Can you work these out from the model? Positions are in its coordinate system, mm. Round coordinates to 2 decimals unless told otherwise and drop trailing zeros. Write each loop counter-clockwise with the first axis right and the second up, starting at its lowest first coordinate (ties: lowest second). Pieces come first, ordered by that corner, then holes. Notation, with made-up numbers: M 62,63 L 120,63 A20 cw 120,70 Z; hole C -2.5,5 d8. An arc over 180 degrees is marked long. Answer as a JSON object with one key per item and string values. Group by question number.
1) Suppose I cut it at A-A, the plane z = 10. Write out the boundary of the cut face in (x, y), and give its area (3 significant figures).
2) I'm going to push flat-ended pins straight in: pin 1 Ø5 at (x, y) = (2, -8) entering from +Z; pin 2 Ø8 at (x, y) = (0.5, 6) entering from -Z; pin 3 Ø12 at (x, y) = (9, -9) entering from +Z. Where does each tip first touch, or does it pass through?
3) Please list where these lines run through material, in increasing order: L1, parallel to Z at x = -11, y = -4; L2, parallel to Z at x = 3.5, y = 7.5; L3, parallel to X at y = 0, z = -7. Write a range as [from, to].
from build123d import *

# Parameters (mm, degrees)
PAD_DEPTH = 15
PAD_TAPER = 40


with BuildPart() as part:
    # Sketch (on XY_Plane of Origin) → Pad (new body, symmetric)
    with BuildSketch(Plane.XY):
        Polygon((0, -15), (12.990381, -7.5), (12.990381, 7.5), (0, 15), (-12.990381, 7.5), (-12.990381, -7.5), align=None)
    extrude(amount=PAD_DEPTH, both=True, taper=PAD_TAPER)


solid = part.part
Results:
{
 "1": {"outline": "M -4.6,-2.66 L 0,-5.31 L 4.6,-2.66 L 4.6,2.66 L 0,5.31 L -4.6,2.66 Z", "area": "73.3 mm^2"},
 "2": {"pin 1": "z = 9.01", "pin 2": "z = -13.38", "pin 3": "z = 7.98"},
 "3": {"L1": "[-2.37, 2.37]", "L2": "[-5.66, 5.66]", "L3": "[-7.12, 7.12]"}
}
